Geometry: final body of the model. Coordinates: model frame, mm. Give positions to 0.01 mm unless a question says otherwise; leave off trailing zeros. Write each loop counter-clockwise with the first axis right and the second up, starting at its lowest first coordinate (ties: lowest second). Pieces come first, ordered by that corner, then holes. Notation, with made-up numbers: (40, -6.5) -> (76, -6.5) arc R11 cw to (76, 7.5) -> close; hole circle Ø9 at (60.25, -11). An arc over 180 degrees is marked (long way). Answer as a JSON object with one key per item and string values.
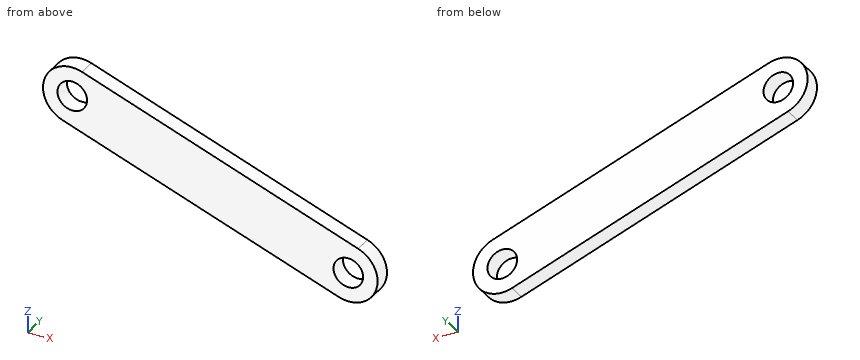
from build123d import *

# Parameters (mm, degrees)
BOSS_EXTRUDE1_DEPTH = 1.27
CUT_EXTRUDE1_REACH  = 4.54
SKETCH3_R           = 2.2479


with BuildPart() as part:
    # Sketch2 → Boss-Extrude1 (new body, symmetric)
    with BuildSketch(Plane(origin=(0, 0, 0), x_dir=(1, 0, 0), z_dir=(0, 1, 0))):
        with BuildLine():
            ThreePointArc((-6.507736872, 31.666944674), (-0.838000837, 28.952143892), (-3.552801619, 23.282407856))
            Line((-3.552801619, 23.282407856), (-45.475485708, 8.507731591))
            ThreePointArc((-45.475485708, 8.507731591), (-51.145221744, 11.222532373), (-48.430420961, 16.892268409))
            Line((-48.430420961, 16.892268409), (-6.507736872, 31.666944674))
        make_face()
    extrude(amount=BOSS_EXTRUDE1_DEPTH, both=True)

    # Sketch3 → Cut-Extrude1 (cut, up to next)
    with BuildSketch(Plane(origin=(0, 1.27, 0), x_dir=(1, 0, 0), z_dir=(0, 1, 0)), mode=Mode.PRIVATE) as cut_extrude1_sk1:
        with Locations((-5.030269245, 27.474676265)):
            Circle(SKETCH3_R)
    cut_extrude1_tool1 = extrude(cut_extrude1_sk1.sketch, amount=-CUT_EXTRUDE1_REACH, mode=Mode.PRIVATE) & part.part
    add(cut_extrude1_tool1.solids().sort_by_distance((-5.030269, 1.27, -27.474676))[0], mode=Mode.SUBTRACT)
    # Sketch3 → Cut-Extrude1 (cut, up to next)
    with BuildSketch(Plane(origin=(0, 1.27, 0), x_dir=(1, 0, 0), z_dir=(0, 1, 0)), mode=Mode.PRIVATE) as cut_extrude1_sk2:
        with Locations((-46.952953335, 12.7)):
            Circle(SKETCH3_R)
    cut_extrude1_tool2 = extrude(cut_extrude1_sk2.sketch, amount=-CUT_EXTRUDE1_REACH, mode=Mode.PRIVATE) & part.part
    add(cut_extrude1_tool2.solids().sort_by_distance((-46.952953, 1.27, -12.7))[0], mode=Mode.SUBTRACT)


solid = part.part
Q1. Material intervals for L1, parallel to Z at x = -46, y = 0.75; L2, parallel to Z at x = -33.5, y = -0.6; L3, parallel to Z at x = -35.5, y = -0.45, sorted ascending. Write a range as from..to.
Values:
{"L1": "-17.75..-14.74, -10.66..-8.36", "L2": "-22.15..-12.73", "L3": "-21.45..-12.02"}
Q2. Cut plane A-A (z = -12.7). Return the cut outline in (x, y), and give its area (3 significant figures).
Values:
{"outline": "(-51.4, -1.27) -> (-49.2, -1.27) -> (-49.2, 1.27) -> (-51.4, 1.27) -> close; (-44.71, -1.27) -> (-33.58, -1.27) -> (-33.58, 1.27) -> (-44.71, 1.27) -> close", "area": "33.8 mm²"}
Q3. First-contact query: P1, Ø1, axis at x = -30, y = -0.5, coming from the +Z side. Flat tip, straight axial feed; report the tip coordinate or a pass-through.
Values:
{"P1": "z = -13.79"}
Q4. Cut plane D-D (z = -20.5). Return the cut outline in (x, y).
Values:
{"outline": "(-38.19, -1.27) -> (-11.45, -1.27) -> (-11.45, 1.27) -> (-38.19, 1.27) -> close"}
Q5. Cut plane C-C (x = -10). Return the cut outline in (y, z), and give its area (3 significant figures).
Values:
{"outline": "(-1.27, -30.44) -> (1.27, -30.44) -> (1.27, -21.01) -> (-1.27, -21.01) -> close", "area": "23.9 mm²"}
Q6. Cut plane B-B (y = 0.4). Return the cut outline in (x, z) (3 decimals).
Values:
{"outline": "(-48.43, -16.892) -> (-6.508, -31.667) arc R4.445 ccw to (-3.553, -23.282) -> (-45.475, -8.508) arc R4.445 ccw to start; hole circle Ø4.496 at (-46.953, -12.7); hole circle Ø4.496 at (-5.03, -27.475)"}
